Source: CAD feature listing. Evaluate the final solid. Frame: model axes, mm. Round coordinates to 2 decimals unless told otherwise and drop trailing zeros. Order: outer loops, then holes, each group sorted by start corner. A loop starts at its lowest first (then second) coordinate and runs counter-clockwise, first axis right, second up. Notation, with made-up numbers: M 16,27 L 43,27 A11 cw 43,40 Z; hole C 67.25,10.25 d11. An arc over 180 degrees is marked long. Answer as CSV lines item,"result". Start each with the question number.
Item 1: Section query C-C on x = -20. Return the cut outline in (y, z), plus the area to 3 significant figures.
Item 2: Section query B-B on y = -46. Return the cut outline in (x, z).
Item 3: Section query A-A on x = -53. Return the cut outline in (y, z), plus the area to 3 significant figures.
Item 4: Line query: line 1 (Y direction, x = 20, z = 6.25); line 2 (X direction, y = -46, z = 8); line 3 (Y direction, x = -93, z = 6.75). Output: solid intervals per line, ascending. Write a range as [from, to].
Item 5: First-contact query: P1, Ø6, axis at x = 53, y = -46, coming from the -Z side; P2, Ø8.5, axis at x = -93, y = 44, coming from the +Z side; P3, Ø7.5, axis at x = -53, y = -46, coming from the +Z side. Flat tips, straight axial feed; report the tip coordinate or a pass-through.
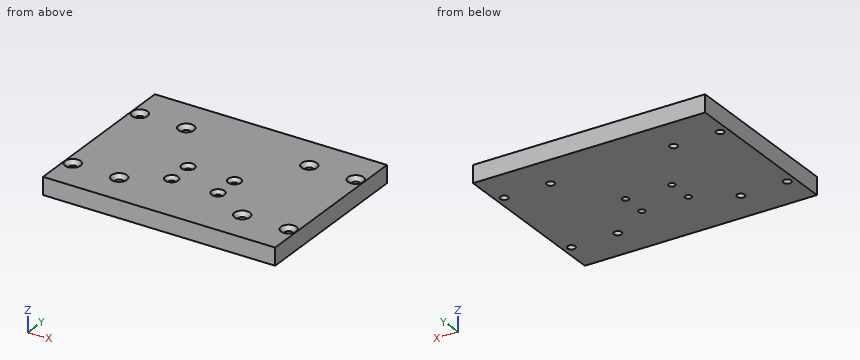
from build123d import *

# Parameters (mm, degrees)
F0_W           = 200
F0_H           = 150
F1_DEPTH       = 15
F3_D           = 6.6
F3_CSINK_D     = 13.44
F3_CSINK_ANGLE = 90
F4_D           = 5.5
F4_CSINK_D     = 11.2
F4_CSINK_ANGLE = 90


with BuildPart() as f1:
    # F0 (on Top) → F1 (new body)
    with BuildSketch(Plane.XY):
        Rectangle(F0_W, F0_H)
    extrude(amount=F1_DEPTH)

    # F3 (through all)
    with Locations(Plane.XY.offset(15)):
        with Locations((-93, 44), (-53, 44), (-93, -46), (-53, -46), (53, 44), (93, 44), (53, -46), (93, -46)):
            CounterSinkHole(F3_D / 2, F3_CSINK_D / 2, counter_sink_angle=F3_CSINK_ANGLE)

    # F4 (through all)
    with Locations(Plane.XY.offset(15)):
        with Locations((-20, -27), (-20, -5), (20, -5), (20, -27)):
            CounterSinkHole(F4_D / 2, F4_CSINK_D / 2, counter_sink_angle=F4_CSINK_ANGLE)


solid = f1.part
Results:
1,outline,"M -75,0 L -29.75,0 L -29.75,12.15 L -32.6,15 L -75,15 Z; M -24.25,0 L -7.75,0 L -7.75,12.15 L -10.6,15 L -21.4,15 L -24.25,12.15 Z; M -2.25,0 L 75,0 L 75,15 L 0.6,15 L -2.25,12.15 Z"
1,area,"2,070 mm^2"
2,outline,"M -100,0 L -96.3,0 L -96.3,11.58 L -99.72,15 L -100,15 Z; M -89.7,0 L -56.3,0 L -56.3,11.58 L -59.72,15 L -86.28,15 L -89.7,11.58 Z; M -49.7,0 L 49.7,0 L 49.7,11.58 L 46.28,15 L -46.28,15 L -49.7,11.58 Z; M 56.3,0 L 89.7,0 L 89.7,11.58 L 86.28,15 L 59.72,15 L 56.3,11.58 Z; M 96.3,0 L 100,0 L 100,15 L 99.72,15 L 96.3,11.58 Z"
3,outline,"M -75,0 L -49.3,0 L -49.3,11.58 L -52.72,15 L -75,15 Z; M -42.7,0 L 40.7,0 L 40.7,11.58 L 37.28,15 L -39.28,15 L -42.7,11.58 Z; M 47.3,0 L 75,0 L 75,15 L 50.72,15 L 47.3,11.58 Z"
3,area,"2,030 mm^2"
4,line 1,"[-75, -29.75], [-24.25, -7.75], [-2.25, 75]"
4,line 2,"[-100, -96.3], [-89.7, -56.3], [-49.7, 49.7], [56.3, 89.7], [96.3, 100]"
4,line 3,"[-75, -49.3], [-42.7, 40.7], [47.3, 75]"
5,P1,"through"
5,P2,"z = 12.53"
5,P3,"z = 12.03"
